Verification items for the finished model (mm, model axes). A direction names the side the tool comes from. Give positions to 0.01 mm unless a question says otherwise; leave off trailing zeros. Write each loop counter-clockwise with the first axis right and the second up, starting at its lowest first coordinate (ties: lowest second). Pieces come first, ordered by that corner, then holes. Notation, with made-up numbers: (-40, -14) -> (-15, -14) arc R18 ccw to (-15, -5) -> close; hole circle Ø4 at (39, 58.25). An arc over 180 degrees is marked (long way). Write item = value, one per line.
from build123d import *


with BuildPart() as part:
    # Szkic1 → Obrót1 (revolve)
    with BuildSketch(Plane.XY, mode=Mode.PRIVATE) as obr_t1_sk:
        Polygon((-62, 0), (-58, 0), (-58, 50), (-62, 50), (-62, 40), (-65, 40), (-65, 10), (-62, 10), align=None)
    revolve(obr_t1_sk.sketch.rotate(Axis((0, 0, 0), (0, 1, 0)), 270), axis=Axis((0, 0, 0), (0, 1, 0)))


solid = part.part
Item 1: Mould release check, pull along X, two halves, no side actions. Record for faces 1 (the cylindrical face through (-61.472, 44.93, 8.071)), 2 (the cylindrical face through (22.21, 25.35, -53.58)), 3 (the flat face through (36, 0, -46)): +X half, -X half, draft (parallel to the pull), parting line (faces both ways), or undercut.
Response values:
face_1 = parting line
face_2 = undercut
face_3 = draft
Item 2: Sectioned sample at C-C on y = 17.5. Record the cut outline in (x, z), then the cut area to 3 significant figures.
Response values:
outline = circle Ø130 at (0, 0); hole circle Ø116 at (0, 0)
area = 2,700 mm^2
Item 3: Sectioned sample at B-B on z = 0. Record the cut outline in (x, y), then the cut area to 3 significant figures.
Response values:
outline = (-65, 10) -> (-62, 10) -> (-62, 0) -> (-58, 0) -> (-58, 50) -> (-62, 50) -> (-62, 40) -> (-65, 40) -> close; (58, 0) -> (62, 0) -> (62, 10) -> (65, 10) -> (65, 40) -> (62, 40) -> (62, 50) -> (58, 50) -> close
area = 580 mm^2
Item 4: Set-up check for faces 4 (the flat face through (23.8, 40, 57.5)), 5 (the flat face through (23.8, 10, -57.5)), 6 (the flat face through (36, 50, 46)): record each of +Z, -Z, +X, -X, +Y, -Y from which the full face is reachable in a straight line by a thin tool's end or side.
Response values:
face_4 = +Y
face_5 = -Y
face_6 = +Z, -Z, +X, -X, +Y
Item 5: Go/stop test with flat-tipped pins: P1, Ø6, axis at x = -36, y = 17.5, coming from the +Z side; P2, Ø8, axis at x = -50, y = 14.5, coming from the +Z side; P3, Ø5, axis at y = 37.5, z = 45, coming from the +X side. Record where each tip stops, or that it passes through.
Response values:
P1 = 56
P2 = 45.92
P3 = 49.18
Item 6: Material ranges on line 1 (X direction, y = 22.5, z = 0); line 2 (Z direction, x = -1, y = 26); line 3 (X direction, y = 4, z = -34), recorded low to high.
Response values:
line_1 = -65 to -58, 58 to 65
line_2 = -64.99 to -57.99, 57.99 to 64.99
line_3 = -51.85 to -46.99, 46.99 to 51.85
Item 7: Sectioned sample at A-A on x = 0. Record the cut outline in (y, z).
Response values:
outline = (0, -62) -> (10, -62) -> (10, -65) -> (40, -65) -> (40, -62) -> (50, -62) -> (50, -58) -> (0, -58) -> close; (0, 58) -> (50, 58) -> (50, 62) -> (40, 62) -> (40, 65) -> (10, 65) -> (10, 62) -> (0, 62) -> close
Item 8: Sectioned sample at D-D on y = 6. Record the cut outline in (x, z), then the cut area to 3 significant figures.
Response values:
outline = circle Ø124 at (0, 0); hole circle Ø116 at (0, 0)
area = 1,510 mm^2
